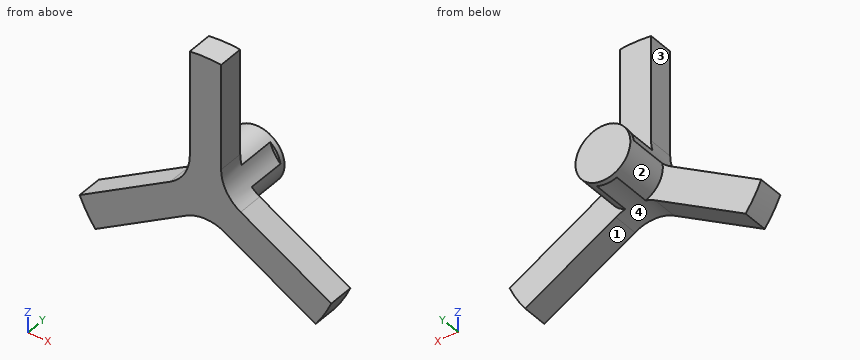
```python
from build123d import *

# Parameters (mm, degrees)
F0_R     = 10.5
F1_DEPTH = 17
F2_R     = 52.5
F3_DEPTH = 10
F5_DEPTH = 25


with BuildPart() as f1:
    # F0 (on Front) → F1 (new body)
    with BuildSketch(Plane.XZ):
        Circle(F0_R)
    extrude(amount=F1_DEPTH)

    # F2 (on face) → F3 (join)
    with BuildSketch(Plane.XZ.offset(17)):
        Circle(F2_R)
    extrude(amount=F3_DEPTH)

    # F4 (on face) → F5 (cut)
    with BuildSketch(Plane.XZ.offset(27)):
        with BuildLine():
            ThreePointArc((-13.5, -0.866025), (-8.009619, 4.624356), (-6, 12.124356))
            Line((-6, 12.124356), (-6, 52.156016))
            ThreePointArc((-6, 52.156016), (-45.466334, 26.25), (-48.168435, -20.881856))
            Line((-48.168435, -20.881856), (-13.5, -0.866025))
        make_face()
        with BuildLine():
            ThreePointArc((52.5, 0), (39.187051, 34.937444), (6, 52.156016))
            Line((6, 52.156016), (6, 12.124356))
            ThreePointArc((6, 12.124356), (8.009619, 4.624356), (13.5, -0.866025))
            Line((13.5, -0.866025), (48.168435, -20.881856))
            ThreePointArc((48.168435, -20.881856), (51.405704, -10.663188), (52.5, 0))
        make_face()
        with BuildLine():
            Line((-7.5, -11.25833), (-42.168435, -31.27416))
            ThreePointArc((-42.168435, -31.27416), (0, -52.5), (42.168435, -31.27416))
            Line((42.168435, -31.27416), (7.5, -11.25833))
            ThreePointArc((7.5, -11.25833), (0, -9.248711), (-7.5, -11.25833))
        make_face()
    extrude(amount=-F5_DEPTH, mode=Mode.SUBTRACT)


solid = f1.part
```
Here's how the part is built. I have some questions about the finished solid (model axes, mm). Face numbers are marked on the shaded views. A direction names the side the tool comes from. Round coordinates to 2 decimals unless told otherwise and drop trailing zeros. Loops run counter-clockwise (first coordinate to the right, second up) from the corner with the lowest first, then second, coordinate; pieces in that order, holes last. Notation, with made-up numbers: (19.5, 77) -> (24.5, 77) arc R9 cw to (24.5, 90) -> close; hole circle Ø2 at (54.25, 18). An arc over 180 degrees is marked (long way). Answer as CSV lines item,"result".
1. If we section it at A-A on z = -26: Please give me the cut outline in (x, y).
Final values:
outline,"(-45.61, -27) -> (-33.03, -27) -> (-33.03, -17) -> (-45.61, -17) -> close; (33.03, -27) -> (45.61, -27) -> (45.61, -17) -> (33.03, -17) -> close"
2. If I drill on L1, parallel to Y at x = 0, z = 13; L2, parallel to X at y = -14.5, z = 9.5; L3, parallel to Z at x = 13.5, y = -18.75, over which ranges is the centre line in solid material (lowest first)?
Final values:
L1,"y = -27 to -17"
L2,"x = -4.47 to 4.47"
L3,"z = -14.72 to -0.87"
3. If we section it at C-C on x = 0: Please give me the cut outline in (y, z), plus the area to 3 significant figures.
Final values:
outline,"(-27, -9.25) -> (-2, -9.25) -> (-2, -10.5) -> (0, -10.5) -> (0, 10.5) -> (-17, 10.5) -> (-17, 52.5) -> (-27, 52.5) -> close"
area,"956 mm^2"
4. For pin 1 (6 mm diameter, centred on x = 31, y = -22, fed in from +Z); pin 2 (1 mm diameter, centred on x = -1.5, z = -10, fed in from -Y); pin 3 (8 mm diameter, centred on y = -23.5, z = 23, fed in from +X), each with a flat end and sliding along its axis, tell me the tip position at first contact or that it passes through.
Final values:
pin 1,"stops at z = -9.24"
pin 2,"stops at y = -2"
pin 3,"stops at x = 6"
5. If we section it at B-B on y = -22.25: Please give me the cut outline in (x, z), plus the area to 3 significant figures.
Final values:
outline,"(-48.17, -20.88) arc R52.5 ccw to (-42.17, -31.27) -> (-7.5, -11.26) arc R15 cw to (7.5, -11.26) -> (42.17, -31.27) arc R52.5 ccw to (48.17, -20.88) -> (13.5, -0.87) arc R15 cw to (6, 12.12) -> (6, 52.16) arc R52.5 ccw to (-6, 52.16) -> (-6, 12.12) arc R15 cw to (-13.5, -0.87) -> close"
area,"1,860 mm^2"
6. If we section it at D-D on z = 39: Please give me the cut outline in (x, y).
Final values:
outline,"(-6, -27) -> (6, -27) -> (6, -17) -> (-6, -17) -> close"
7. Which directions (+Z, -Z, +X, -X, +Y, -Y) give clear straight access to the entire face, cutting with the end or side of a thin tool? Please do the marked faces 1, 2, 3 and 4.
Final values:
face 1,"-Z, +Y, -Y"
face 2,"+Y"
face 3,"+Z, -X, +Y, -Y"
face 4,"-Z, -Y"
